For this review, use the dimensioned drawing (mm, ordinates from the lowest corner) and the shaded views. Round coordinates to 2 decimals unless told otherwise and drop trailing zeros. Order: outer loops, then holes, each group sorted by start corner. A loop starts at its lowest first (then second) coordinate and runs counter-clockwise, first axis right, second up. Notation, with made-up numbers: M -10.5,2 L 24.5,2 A22 ccw 24.5,8 Z; hole C 11,49.5 d10. An arc over 180 degrees is marked long. One line per item, written item: value. Start each with the question number.
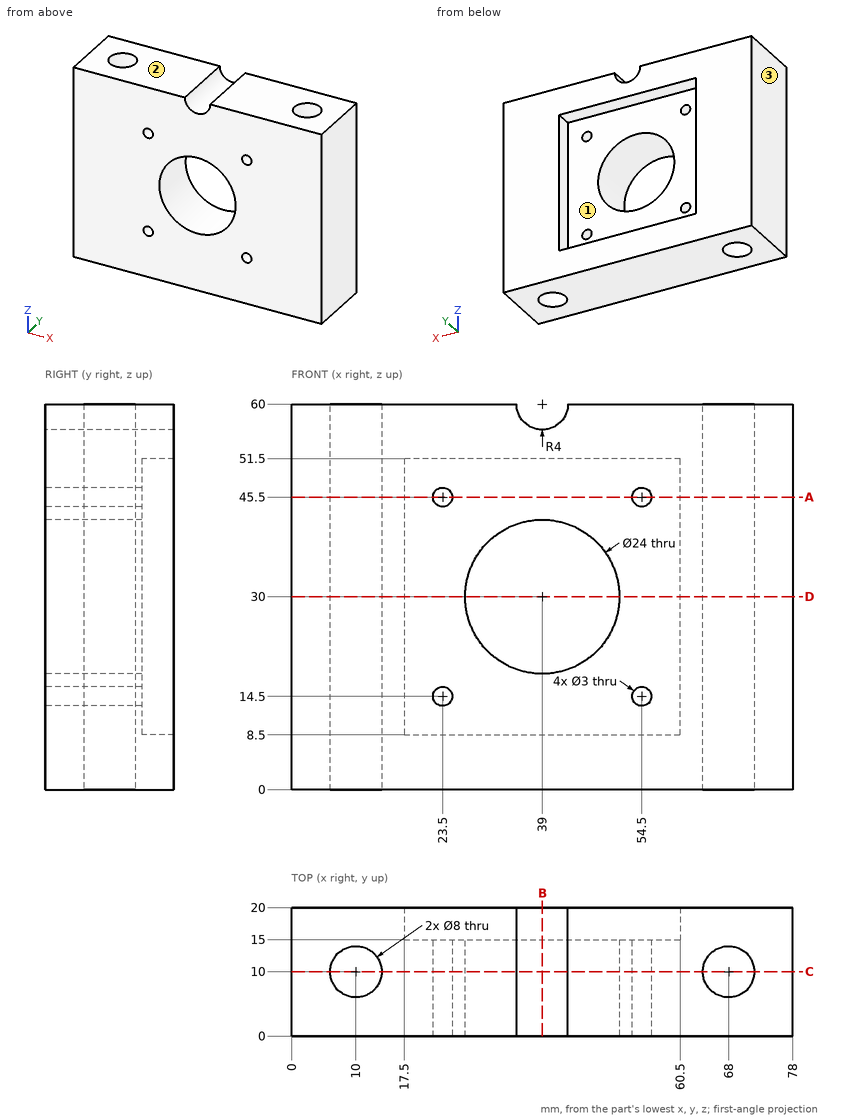
Item 1: Consider section C-C, the plane y = 10. Give the boundary of the cut face in (x, z).
Item 2: Consider section D-D, the plane z = 30. Give the boundary of the cut face in (x, y), then the cut area to 3 significant figures.
Item 3: Wall thickness on L1, parallel to Z at x = 54.5, y = 11; L2, parallel to X at y = 15.75, z = 29.5; L3, parallel to Y at x = 10, z = 38: over which ranges is each line inside the solid? List them lowest first.
Item 4: Clearance check with flat-ended pins moving along their axes: P1, Ø6.5, axis at x = 68, y = 10, coming from the +Z side; P2, Ø1.5, axis at x = 40, y = 18.5, coming from the +Z side. State where each tip first meets the part, or that it passes through.
Item 5: Consider section A-A, the plane z = 45.5. Give the boundary of the cut face in (x, y).
Item 6: The part is to be moulded in two halves that separate along Z. For the marked faces 1, 2 and 3, say which applies: pulls with the +Z half, pulls with the -Z half, needs draft (parallel to the pull), parting line crosses it, or undercut.
Item 7: Consider section B-B, the plane x = 39. Give the boundary of the cut face in (y, z).
Computed:
1. outline: M 0,0 L 6,0 L 6,60 L 0,60 Z; M 14,0 L 64,0 L 64,60 L 43,60 A4 cw 35,60 L 14,60 Z; M 72,0 L 78,0 L 78,60 L 72,60 Z; hole C 23.5,14.5 d3; hole C 23.5,45.5 d3; hole C 39,30 d24; hole C 54.5,14.5 d3; hole C 54.5,45.5 d3
2. outline: M 0,0 L 27,0 L 27,15 L 17.5,15 L 17.5,20 L 0,20 Z; M 51,0 L 78,0 L 78,20 L 60.5,20 L 60.5,15 L 51,15 Z; hole C 10,10 d8; hole C 68,10 d8
2. area: 884 mm^2
3. L1: z = 0 to 13, 16 to 44, 47 to 60
3. L2: x = 0 to 17.5, 60.5 to 78
3. L3: y = 0 to 6, 14 to 20
4. P1: passes through
4. P2: stops at z = 56.4
5. outline: M 0,0 L 22,0 L 22,15 L 17.5,15 L 17.5,20 L 0,20 Z; M 25,0 L 53,0 L 53,15 L 25,15 Z; M 56,0 L 78,0 L 78,20 L 60.5,20 L 60.5,15 L 56,15 Z; hole C 10,10 d8; hole C 68,10 d8
6. face 1: undercut
6. face 2: pulls with the +Z half
6. face 3: needs draft
7. outline: M 0,0 L 20,0 L 20,8.5 L 15,8.5 L 15,18 L 0,18 Z; M 0,42 L 15,42 L 15,51.5 L 20,51.5 L 20,56 L 0,56 Z
